Read the model definition and answer for the solid it produces. Units are mm, in the model's axes. Face numbers are marked on the shaded views. A direction names the side the tool comes from. Give positions to 0.01 mm unless a question says otherwise; leave off trailing zeros. Loops run counter-clockwise (first coordinate to the right, second up) from the corner with the lowest first, then second, coordinate; pieces in that order, holes last. Notation, with made-up numbers: (22.25, 4.5) - (33.25, 4.5) arc R29 ccw to (33.25, 34.5) - close; hole circle Ø5 at (8.25, 60). An arc over 180 degrees is marked (long way). Write item = value, one per line. Start each with the question number.
from build123d import *

# Parameters (mm, degrees)
SKETCH3_W           = 70
SKETCH3_H           = 40
BOSS_EXTRUDE2_DEPTH = 70
SKETCH4_W           = 65
SKETCH4_H           = 35
CUT_EXTRUDE1_DEPTH  = 71
SKETCH5_W           = 12.5
SKETCH5_H           = 70
BOSS_EXTRUDE3_DEPTH = 10


with BuildPart() as part:
    # Sketch3 → Boss-Extrude2 (new body)
    with BuildSketch(Plane(origin=(0, 0, 0), x_dir=(1, 0, 0), z_dir=(0, 1, 0))):
        Rectangle(SKETCH3_W, SKETCH3_H)
    extrude(amount=BOSS_EXTRUDE2_DEPTH)

    # Sketch4 → Cut-Extrude1 (cut, through all)
    with BuildSketch(Plane(origin=(0, 70, 0), x_dir=(1, 0, 0), z_dir=(0, 1, 0))):
        Rectangle(SKETCH4_W, SKETCH4_H)
    extrude(amount=-CUT_EXTRUDE1_DEPTH, mode=Mode.SUBTRACT)

    # Sketch5 → Boss-Extrude3 (add)
    with BuildSketch(Plane(origin=(-32.5, 0, 0), x_dir=(0, 0, -1), z_dir=(1, 0, 0))):
        with Locations((-11.25, 35)):
            Rectangle(SKETCH5_W, SKETCH5_H)
        with Locations((11.25, 35)):
            Rectangle(SKETCH5_W, SKETCH5_H)
    boss_extrude3 = extrude(amount=BOSS_EXTRUDE3_DEPTH)

    # Mirror1: Boss-Extrude3 across plane
    add(boss_extrude3.mirror(Plane(origin=(0, 0, 0), x_dir=(0, 0, 1), z_dir=(1, 0, 0))))


solid = part.part
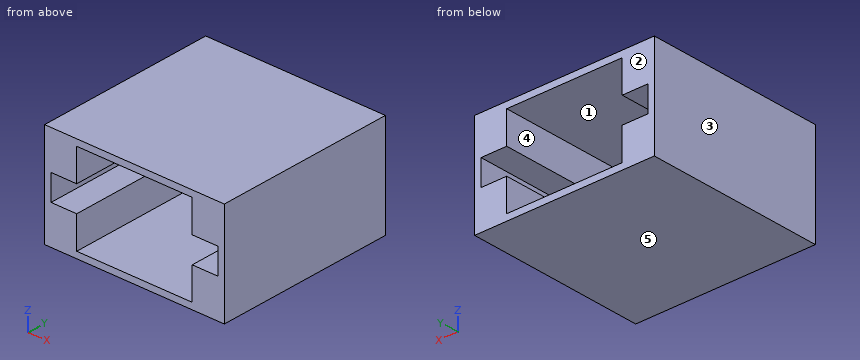
1. A tool of negligible diameter and unlimited length cuts with its end or side. For the marked faces 4 and 5, from which of +Z, -Z, +X, -X, +Y, -Y can it reach the whole face along a straight path? Write none if from no direction.
2. A cutting plane is placed at C-C on y = 7.5. Give the vertices of the cut face in (x, z).
3. A cutting plane is placed at A-A on z = 4. Give the vertices of the cut face in (x, y).
4. Given P1, Ø2, axis at x = -20.5, z = -15.5, coming from the -Y side, flat-ended and moving along its own axis, determine where the tip first touches the part or whether it passes through.
5. For a pull along X with two mould halves and no side action, classify the marked faces 1, 2 and 3 as released by +X, released by -X, zero draft, split by the parting line, or undercut.
6. Consider line 1 along X through (y, z) = (52, 14.5); line 2 along X through (y, z) = (23.5, -3.5); line 3 along Z through (x, y) = (-15, 50.5). Determine where each line is inside the solid, lowest interval first. Write a range as [from, to].
7. A cutting plane is placed at B-B on x = -31. Give the vertices of the cut face in (y, z), and give its area (3 significant figures).
Reply:
q1.face_4 = +Y, -Y
q1.face_5 = -Z, +X, -X, +Y, -Y
q2.outline = (-35, -20) - (35, -20) - (35, 20) - (-35, 20) - close; hole (-32.5, -5) - (-22.5, -5) - (-22.5, -17.5) - (22.5, -17.5) - (22.5, -5) - (32.5, -5) - (32.5, 5) - (22.5, 5) - (22.5, 17.5) - (-22.5, 17.5) - (-22.5, 5) - (-32.5, 5) - close
q3.outline = (-35, 0) - (-32.5, 0) - (-32.5, 70) - (-35, 70) - close; (32.5, 0) - (35, 0) - (35, 70) - (32.5, 70) - close
q4.P1 = through
q5.face_1 = undercut
q5.face_2 = zero draft
q5.face_3 = released by -X
q6.line_1 = [-35, -22.5], [22.5, 35]
q6.line_2 = [-35, -32.5], [32.5, 35]
q6.line_3 = [-20, -17.5], [17.5, 20]
q7.outline = (0, -20) - (70, -20) - (70, -5) - (0, -5) - close; (0, 5) - (70, 5) - (70, 20) - (0, 20) - close
q7.area = 2,100 mm^2
